Geometry: see drawing. Coordinates: mm, zero at the bounding-box minimum. Round coordinates to 2 decimals unless told otherwise and drop trailing zeros. Write each loop counter-clockwise with the first axis right and the second up, starting at its lowest first coordinate (ties: lowest second). Pieces come first, ordered by that corner, then holes. Notation, with made-up numbers: (88, 13) -> (95, 13) arc R13 cw to (95, 30) -> close; hole circle Ø1 at (-12.5, -24). An arc over 180 degrees is marked (long way). Use CSV: the item, a comma, the result in double quotes.
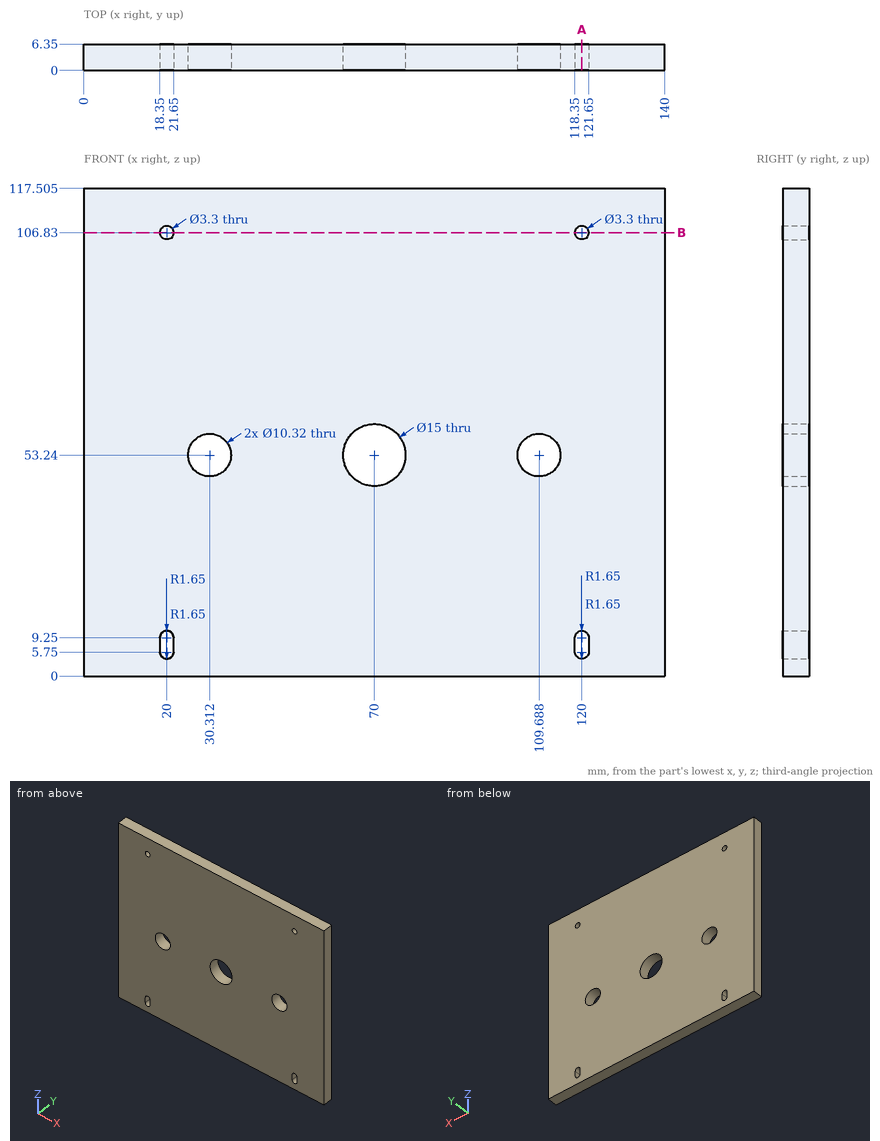
Item 1: Section query B-B on z = 106.83. Return the cut outline in (x, y).
Worked answers:
outline,"(0, 0) -> (18.35, 0) -> (18.35, 6.35) -> (0, 6.35) -> close; (21.65, 0) -> (118.35, 0) -> (118.35, 6.35) -> (21.65, 6.35) -> close; (121.65, 0) -> (140, 0) -> (140, 6.35) -> (121.65, 6.35) -> close"
Item 2: Section query A-A on x = 120. Give the number of separate pieces and of enclosed holes in the cut face, plus the area to 3 significant figures.
Worked answers:
separate pieces,"3"
enclosed holes,"0"
area,"682 mm²"
Item 3: Line query: line 1 (X direction, y = 2.25, z = 107); line 2 (X direction, y = 2.75, z = 53.24); line 3 (Z direction, x = 20, y = 1.5) (1 decimal). Output: solid intervals per line, ascending.
Worked answers:
line 1,"x = 0 to 18.36, 21.64 to 118.36, 121.64 to 140"
line 2,"x = 0 to 25.15, 35.47 to 62.5, 77.5 to 104.53, 114.85 to 140"
line 3,"z = 0 to 4.1, 10.9 to 105.2, 108.5 to 117.5"
